Geometry check sheet. Reference: the model listing, model coordinates, mm. Face numbers are marked on the shaded views. Round coordinates to 2 decimals unless told otherwise and drop trailing zeros. Write each loop counter-clockwise with the first axis right and the second up, starting at its lowest first coordinate (ties: lowest second). Pieces come first, ordered by that corner, then holes.
Item 1: Draft check along X on the marked faces 1 and 2. Enter one of: pulls with the +X half, pulls with the -X half, needs draft (parallel to the pull), parting line crosses it, or undercut.
Item 2: Cross-section at B-B (x = 41.5). Enter the section's corners in (y, z).
Item 3: Scan lines: probe 1 along X at (y, z) = (71, 4.75); probe 2 along Y at (x, z) = (70.62, 5.3); probe 3 along Y at (x, z) = (42, 6.25). Record each from-to range of solid material in increasing order.
Item 4: Cross-section at C-C (x = 70.62). State how many separate pieces and enclosed holes the cut face has, then the cut area to 3 significant figures.
Item 5: Depth check by flat-ended pin: P1, Ø1.6, axis at y = 33, z = 7, coming from the -X side; P2, Ø5.5, axis at x = 4.38, y = 4.22, coming from the -Z side; P3, Ø1, axis at x = 32, y = 37.5, coming from the +Z side. Enter the tip coordinate at first touch or a pass-through.
Item 6: Cross-section at A-A (y = 69.5). Enter the section's corners in (x, z).
from build123d import *

# Parameters (mm, degrees)
BOX003_W          = 77
BOX003_H          = 87
BOX003_DEPTH      = 10
BOX002_W          = 79
BOX002_H          = 89
BOX002_DEPTH      = 10
CYLINDER005_R     = 1.75
CYLINDER005_DEPTH = 10
CYLINDER006_R     = 1.75
CYLINDER006_DEPTH = 10
CYLINDER007_R     = 1.75
CYLINDER007_DEPTH = 10
CYLINDER008_R     = 1.75
CYLINDER008_DEPTH = 10
PRISM_DEPTH       = 4
PRISM001_DEPTH    = 4
PRISM002_DEPTH    = 4
PRISM003_DEPTH    = 4
CYLINDER_R        = 1.75
CYLINDER_DEPTH    = 10
CYLINDER001_R     = 1.75
CYLINDER001_DEPTH = 10
CYLINDER002_R     = 1.75
CYLINDER002_DEPTH = 10
CYLINDER003_R     = 1.75
CYLINDER003_DEPTH = 10
BOX_W             = 75
BOX_H             = 85
BOX_DEPTH         = 10
BOX001_W          = 79
BOX001_H          = 89
BOX001_DEPTH      = 8
CYLINDER011_R     = 4
CYLINDER011_DEPTH = 4
CYLINDER010_R     = 4
CYLINDER010_DEPTH = 4
CYLINDER009_R     = 4
CYLINDER009_DEPTH = 4
CYLINDER004_R     = 4
CYLINDER004_DEPTH = 4
FILLET001_R       = 2
BOX005_W          = 15
BOX005_H          = 5
BOX005_DEPTH      = 6
BOX006_W          = 5
BOX006_H          = 89
BOX006_DEPTH      = 6
BOX004_W          = 15
BOX004_H          = 5
BOX004_DEPTH      = 6
FILLET_R          = 2


with BuildPart() as cube003:
    # Box003 → Box003 (new body)
    with BuildSketch(Plane(origin=(-1, -1, 10), x_dir=(1, 0, 0), z_dir=(0, 0, 1))):
        with Locations((38.5, 43.5)):
            Rectangle(BOX003_W, BOX003_H)
    extrude(amount=BOX003_DEPTH)


with BuildPart() as cut013:
    # Box002 → Box002 (new body)
    with BuildSketch(Plane(origin=(-2, -2, 10), x_dir=(1, 0, 0), z_dir=(0, 0, 1))):
        with Locations((39.5, 44.5)):
            Rectangle(BOX002_W, BOX002_H)
    extrude(amount=BOX002_DEPTH)

    # Cut013: cut Cube003
    add(cube003.part, mode=Mode.SUBTRACT)


with BuildPart() as cut013_1:
    # Cut013 placement: moved
    add(cut013.part.moved(Location((0, 0, -4))))


with BuildPart() as cylinder005:
    # Cylinder005 → Cylinder005 (new body)
    with BuildSketch(Plane(origin=(4.38, 4.22, -1), x_dir=(1, 0, 0), z_dir=(0, 0, 1))):
        Circle(CYLINDER005_R)
    extrude(amount=CYLINDER005_DEPTH)


with BuildPart() as cylinder006:
    # Cylinder006 → Cylinder006 (new body)
    with BuildSketch(Plane(origin=(70.62, 4.22, -1), x_dir=(1, 0, 0), z_dir=(0, 0, 1))):
        Circle(CYLINDER006_R)
    extrude(amount=CYLINDER006_DEPTH)


with BuildPart() as cylinder007:
    # Cylinder007 → Cylinder007 (new body)
    with BuildSketch(Plane(origin=(70.62, 80.78, -1), x_dir=(1, 0, 0), z_dir=(0, 0, 1))):
        Circle(CYLINDER007_R)
    extrude(amount=CYLINDER007_DEPTH)


with BuildPart() as cylinder008:
    # Cylinder008 → Cylinder008 (new body)
    with BuildSketch(Plane(origin=(4.38, 80.78, -1), x_dir=(1, 0, 0), z_dir=(0, 0, 1))):
        Circle(CYLINDER008_R)
    extrude(amount=CYLINDER008_DEPTH)


with BuildPart() as prism:
    # Prism → Prism (new body)
    with BuildSketch(Plane(origin=(4.38, 4.22, 0), x_dir=(1, 0, 0), z_dir=(0, 0, 1))):
        Polygon((3.5, 0), (1.75, 3.031089), (-1.75, 3.031089), (-3.5, 0), (-1.75, -3.031089), (1.75, -3.031089), align=None)
    extrude(amount=PRISM_DEPTH)


with BuildPart() as prism001:
    # Prism001 → Prism001 (new body)
    with BuildSketch(Plane(origin=(70.62, 4.22, 0), x_dir=(1, 0, 0), z_dir=(0, 0, 1))):
        Polygon((3.5, 0), (1.75, 3.031089), (-1.75, 3.031089), (-3.5, 0), (-1.75, -3.031089), (1.75, -3.031089), align=None)
    extrude(amount=PRISM001_DEPTH)


with BuildPart() as prism002:
    # Prism002 → Prism002 (new body)
    with BuildSketch(Plane(origin=(70.62, 80.78, 0), x_dir=(1, 0, 0), z_dir=(0, 0, 1))):
        Polygon((3.5, 0), (1.75, 3.031089), (-1.75, 3.031089), (-3.5, 0), (-1.75, -3.031089), (1.75, -3.031089), align=None)
    extrude(amount=PRISM002_DEPTH)


with BuildPart() as prism003:
    # Prism003 → Prism003 (new body)
    with BuildSketch(Plane(origin=(4.38, 80.78, 0), x_dir=(1, 0, 0), z_dir=(0, 0, 1))):
        Polygon((3.5, 0), (1.75, 3.031089), (-1.75, 3.031089), (-3.5, 0), (-1.75, -3.031089), (1.75, -3.031089), align=None)
    extrude(amount=PRISM003_DEPTH)


with BuildPart() as cylinder:
    # Cylinder → Cylinder (new body)
    with BuildSketch(Plane(origin=(4.38, 80.78, 0), x_dir=(1, 0, 0), z_dir=(0, 0, 1))):
        Circle(CYLINDER_R)
    extrude(amount=CYLINDER_DEPTH)


with BuildPart() as cylinder001:
    # Cylinder001 → Cylinder001 (new body)
    with BuildSketch(Plane(origin=(70.62, 80.78, 0), x_dir=(1, 0, 0), z_dir=(0, 0, 1))):
        Circle(CYLINDER001_R)
    extrude(amount=CYLINDER001_DEPTH)


with BuildPart() as cylinder002:
    # Cylinder002 → Cylinder002 (new body)
    with BuildSketch(Plane(origin=(70.62, 4.22, 0), x_dir=(1, 0, 0), z_dir=(0, 0, 1))):
        Circle(CYLINDER002_R)
    extrude(amount=CYLINDER002_DEPTH)


with BuildPart() as cylinder003:
    # Cylinder003 → Cylinder003 (new body)
    with BuildSketch(Plane(origin=(4.38, 4.22, 0), x_dir=(1, 0, 0), z_dir=(0, 0, 1))):
        Circle(CYLINDER003_R)
    extrude(amount=CYLINDER003_DEPTH)


with BuildPart() as cube:
    # Box → Box (new body)
    with BuildSketch(Plane.XY.offset(2)):
        with Locations((37.5, 42.5)):
            Rectangle(BOX_W, BOX_H)
    extrude(amount=BOX_DEPTH)


with BuildPart() as cut004:
    # Box001 → Box001 (new body)
    with BuildSketch(Plane(origin=(-2, -2, 0), x_dir=(1, 0, 0), z_dir=(0, 0, 1))):
        with Locations((39.5, 44.5)):
            Rectangle(BOX001_W, BOX001_H)
    extrude(amount=BOX001_DEPTH)

    # Cut: cut Cube
    add(cube.part, mode=Mode.SUBTRACT)

    # Cut001: cut Cylinder003
    add(cylinder003.part, mode=Mode.SUBTRACT)

    # Cut002: cut Cylinder002
    add(cylinder002.part, mode=Mode.SUBTRACT)

    # Cut003: cut Cylinder001
    add(cylinder001.part, mode=Mode.SUBTRACT)

    # Cut004: cut Cylinder
    add(cylinder.part, mode=Mode.SUBTRACT)


with BuildPart() as fusion:
    # Cylinder011 → Cylinder011 (new body)
    with BuildSketch(Plane(origin=(4.38, 80.78, 2), x_dir=(1, 0, 0), z_dir=(0, 0, 1))):
        Circle(CYLINDER011_R)
    extrude(amount=CYLINDER011_DEPTH)

    # Fusion: union Cut004
    add(cut004.part)


with BuildPart() as fusion001:
    # Cylinder010 → Cylinder010 (new body)
    with BuildSketch(Plane(origin=(70.62, 80.78, 2), x_dir=(1, 0, 0), z_dir=(0, 0, 1))):
        Circle(CYLINDER010_R)
    extrude(amount=CYLINDER010_DEPTH)

    # Fusion001: union Fusion
    add(fusion.part)


with BuildPart() as fusion002:
    # Cylinder009 → Cylinder009 (new body)
    with BuildSketch(Plane(origin=(70.62, 4.22, 2), x_dir=(1, 0, 0), z_dir=(0, 0, 1))):
        Circle(CYLINDER009_R)
    extrude(amount=CYLINDER009_DEPTH)

    # Fusion002: union Fusion001
    add(fusion001.part)


with BuildPart() as fillet001:
    # Cylinder004 → Cylinder004 (new body)
    with BuildSketch(Plane(origin=(4.38, 4.22, 2), x_dir=(1, 0, 0), z_dir=(0, 0, 1))):
        Circle(CYLINDER004_R)
    extrude(amount=CYLINDER004_DEPTH)

    # Fusion003: union Fusion002
    add(fusion002.part)

    # Cut005: cut Prism003
    add(prism003.part, mode=Mode.SUBTRACT)

    # Cut006: cut Prism002
    add(prism002.part, mode=Mode.SUBTRACT)

    # Cut007: cut Prism001
    add(prism001.part, mode=Mode.SUBTRACT)

    # Cut008: cut Prism
    add(prism.part, mode=Mode.SUBTRACT)

    # Cut009: cut Cylinder008
    add(cylinder008.part, mode=Mode.SUBTRACT)

    # Cut010: cut Cylinder007
    add(cylinder007.part, mode=Mode.SUBTRACT)

    # Cut011: cut Cylinder006
    add(cylinder006.part, mode=Mode.SUBTRACT)

    # Cut012: cut Cylinder005
    add(cylinder005.part, mode=Mode.SUBTRACT)

    # Cut014: cut Cut013
    add(cut013_1.part, mode=Mode.SUBTRACT)

    # Fillet001
    fillet001_edges = [fillet001.edges().sort_by_distance(p)[0] for p in [
        (-2, 42.5, 0),
        (37.5, 87, 0),
        (37.5, -2, 0),
    ]]
    fillet(fillet001_edges, radius=FILLET001_R)


with BuildPart() as cube005:
    # Box005 → Box005 (new body)
    with BuildSketch(Plane(origin=(77, 82, 0), x_dir=(1, 0, 0), z_dir=(0, 0, 1))):
        with Locations((7.5, 2.5)):
            Rectangle(BOX005_W, BOX005_H)
    extrude(amount=BOX005_DEPTH)


with BuildPart() as cube006:
    # Box006 → Box006 (new body)
    with BuildSketch(Plane(origin=(92, -2, 0), x_dir=(1, 0, 0), z_dir=(0, 0, 1))):
        with Locations((2.5, 44.5)):
            Rectangle(BOX006_W, BOX006_H)
    extrude(amount=BOX006_DEPTH)


with BuildPart() as fusion005:
    # Box004 → Box004 (new body)
    with BuildSketch(Plane(origin=(77, -2, 0), x_dir=(1, 0, 0), z_dir=(0, 0, 1))):
        with Locations((7.5, 2.5)):
            Rectangle(BOX004_W, BOX004_H)
    extrude(amount=BOX004_DEPTH)

    # Fusion004: union Cube005, Cube006
    add(cube005.part)
    add(cube006.part)

    # Fillet
    fillet_edges = [fusion005.edges().sort_by_distance(p)[0] for p in [
        (84.5, -2, 0),
        (97, 42.5, 0),
        (84.5, 87, 0),
    ]]
    fillet(fillet_edges, radius=FILLET_R)

    # Fusion005: union Fillet001
    add(fillet001.part)


solid = fusion005.part
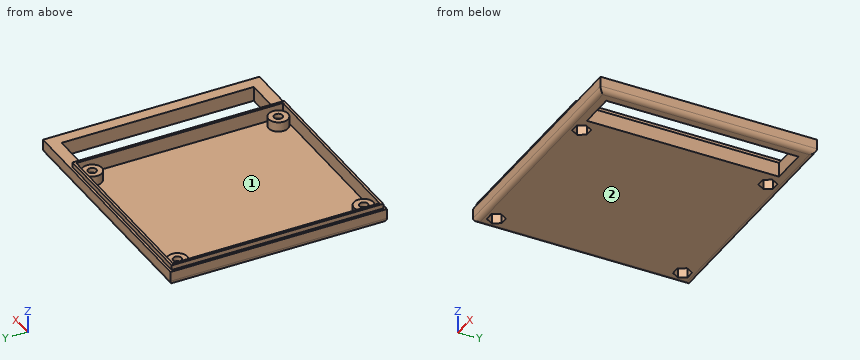
Resolved:
1. face 1: undercut
1. face 2: needs draft
2. outline: (-2, 2) arc R2 ccw to (0, 0) - (85, 0) arc R2 ccw to (87, 2) - (87, 6) - (86, 6) - (86, 8) - (85, 8) - (85, 2) - (0, 2) - (0, 8) - (-1, 8) - (-1, 6) - (-2, 6) - close
3. probe 1: x = -2 to 0, 75 to 77, 92 to 97
3. probe 2: y = -2 to 0, 0.22 to 2.47, 5.97 to 8.22, 76.78 to 79.03, 82.53 to 84.78, 85 to 87
3. probe 3: y = -1 to 0, 85 to 86
4. separate pieces: 3
4. enclosed holes: 0
4. area: 198 mm2
5. P1: stops at x = -1
5. P2: stops at z = 4
5. P3: stops at z = 2
6. outline: (-2, 2) arc R2 ccw to (0, 0) - (77, 0) - (77, 6) - (76, 6) - (76, 8) - (75, 8) - (75, 2) - (0, 2) - (0, 8) - (-1, 8) - (-1, 6) - (-2, 6) - close; (92, 0) - (95, 0) arc R2 ccw to (97, 2) - (97, 6) - (92, 6) - close
